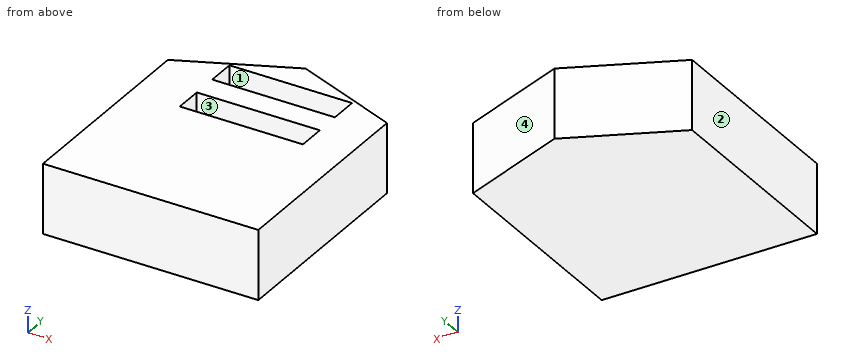
```python
from build123d import *

# Parameters (mm, degrees)
F0_W     = 129.2205303907
F0_H     = 41.7168587446
F1_DEPTH = 152.4
F2_W     = 73.6317485571
F2_H     = 16.954690218
F2_W_2   = 73.8739818335
F2_H_2   = 16.7124718428
F3_DEPTH = 25.4
F5_DEPTH = 41.7178587446


with BuildPart() as f1:
    # F0 (on Front) → F1 (new body)
    with BuildSketch(Plane.XZ):
        with Locations((-0.3052428365, -6.4101442695)):
            Rectangle(F0_W, F0_H)
    extrude(amount=F1_DEPTH)

    # F2 (on face) → F3 (cut)
    with BuildSketch(Plane.XY.offset(14.4482851028)):
        with Locations((1.6954615712, -25.9895175695)):
            Rectangle(F2_W, F2_H)
        with Locations((1.8165782094, -58.0823048949)):
            Rectangle(F2_W_2, F2_H_2)
    extrude(amount=-F3_DEPTH, mode=Mode.SUBTRACT)

    # F4 (on face) → F5 (cut, through all)
    with BuildSketch(Plane.XY.offset(14.4482851028)):
        Polygon((64.3050223589, 0), (0, 0), (64.3050223589, -25.4777166992), align=None)
        Polygon((-64.9155080318, 0), (-64.9155080318, -29.2058624327), (0, 0), align=None)
    extrude(amount=-F5_DEPTH, mode=Mode.SUBTRACT)


solid = f1.part
```
Geometry check sheet. Reference: the model listing, model coordinates, mm. Face numbers are marked on the shaded views. Give positions to 0.01 mm unless a question says otherwise; leave off trailing zeros. Write each loop counter-clockwise with the first axis right and the second up, starting at its lowest first coordinate (ties: lowest second). Pieces come first, ordered by that corner, then holes.
1) Section check B-B, the plane x = -20. Record the boundary of the cut face in (y, z).
2) Section check A-A, the plane z = 9. Record the boundary of the cut face in (x, y), and give its area (3 significant figures).
3) Release check for a two-part mould opening along Y. For the marked faces 1, 2, 3 and 4 record: pulls with the +Y half, pulls with the -Y half, needs draft (parallel to the pull), parting line crosses it, or undercut.
4) Section check C-C, the plane y = -63. Record the boundary of the cut face in (x, z), and give its area (3 significant figures).
5) Section check D-D, the plane z = -16.5. Record the boundary of the cut face in (x, y), and give its area (3 significant figures).
6) Material ranges on L1, parallel to Z at x = -8, y = -63.5; L2, parallel to Y at x = -38, z = 10; L3, parallel to Y at x = -14.5, z = -19, recorded low to high.
7) Gauge pin test, flat ends, axial feed: pin 1 (5 mm diameter, centred on y = -23.5, z = 2.5, fed in from -X); pin 2 (3 mm diameter, centred on y = -18.5, z = 6, fed in from -X); pin 3 (20.5 mm diameter, centred on x = 19.5, z = 6.5, fed in from +Y). Record the tip position at first contact, or that the pin passes through.
Computed:
1. outline: (-152.4, -27.27) - (-9, -27.27) - (-9, 14.45) - (-17.51, 14.45) - (-17.51, -10.95) - (-34.47, -10.95) - (-34.47, 14.45) - (-49.73, 14.45) - (-49.73, -10.95) - (-66.44, -10.95) - (-66.44, 14.45) - (-152.4, 14.45) - close
2. outline: (-64.92, -152.4) - (64.31, -152.4) - (64.31, -25.48) - (0, 0) - (-64.92, -29.21) - close; hole (-35.12, -66.44) - (38.75, -66.44) - (38.75, -49.73) - (-35.12, -49.73) - close; hole (-35.12, -34.47) - (38.51, -34.47) - (38.51, -17.51) - (-35.12, -17.51) - close
2. area: 15,400 mm2
3. face 1: undercut
3. face 2: needs draft
3. face 3: undercut
3. face 4: pulls with the +Y half
4. outline: (-64.92, -27.27) - (64.31, -27.27) - (64.31, 14.45) - (38.75, 14.45) - (38.75, -10.95) - (-35.12, -10.95) - (-35.12, 14.45) - (-64.92, 14.45) - close
4. area: 3,510 mm2
5. outline: (-64.92, -152.4) - (64.31, -152.4) - (64.31, -25.48) - (0, 0) - (-64.92, -29.21) - close
5. area: 17,900 mm2
6. L1: z = -27.27 to -10.95
6. L2: y = -152.4 to -17.1
6. L3: y = -152.4 to -6.52
7. pin 1: stops at x = -57.79
7. pin 2: stops at x = -44.45
7. pin 3: stops at y = -3.66
